Here's how the part is built. I have some questions about the finished solid (model axes, mm). A direction names the side the tool comes from. Coordinates: 2 decimals unless noted, no trailing zeros. Loops run counter-clockwise (first coordinate to the right, second up) from the corner with the lowest first, then second, coordinate; pieces in that order, holes last. Notation, with made-up numbers: M 14.25,75 L 19.25,75 A26 cw 19.25,93 Z; hole C 11,16.25 d4. An arc over 180 degrees is marked long. Use CSV: the item, a comma, the result in double quotes. Start each with the question number.
Q1. If we section it at A-A (x = -9): Please give me the cut outline in (y, z).
Q2. If we section it at C-C (y = 4.25): Please give me the cut outline in (x, z).
Q3. If we mould it in two halves opening along X, with no side actions, what happens to faces 1 (the cylindrical face through (-70.885, 26.549, -133.04)), 2 (the flat face through (-80, 15, -69)), 3 (the flat face through (-39, 27.5, -71))? For each: +X half, -X half, draft (parallel to the pull), parting line (faces both ways), or undercut.
Q4. Please list where these lines run through material, in increasing order: probe 1 along Y at (x, z) = (-46.5, -73); probe 2 along X at (y, z) = (25, -132.5); probe 3 along Z at (x, y) = (-9.5, 13). Write a range as [from, to].
Q5. For pin 1 Ø12 at (y, z) = (13.5, -49.5) entering from +X; pin 2 Ø2.5 at (x, z) = (-74.5, -131) entering from +Y, each with a flat end and sliding along its axis, tell me the tip position at first contact or that it passes through.
Q6. If we section it at D-D (x = -75): Please give me the cut outline in (y, z).
Q7. Which directions (+Z, -Z, +X, -X, +Y, -Y) give clear straight access to the entire face, cutting with the end or side of a thin tool? Please do faces 4 (the flat face through (-38, 15, -137.5)), 5 (the flat face through (-40, 30, -71)), 6 (the flat face through (-75, 23, -8)).
Q8. If we section it at B-B (z = -132.5): Please give me the cut outline in (x, y), and give its area (3 significant figures).
from build123d import *

# Parameters (mm, degrees)
SKETCH1_W           = 81
SKETCH1_H           = 140
BOSS_EXTRUDE2_DEPTH = 30
SKETCH3_R           = 4.15
CUT_EXTRUDE2_DEPTH  = 7
SHELL1_START        = 2.5
SHELL1_DEPTH        = 25
SHELL1_2_DEPTH      = 18


# Read off the part's stored shape, not the designer's step: Shell1
with BuildPart() as part:
    # Sketch1 → Boss-Extrude2 (new body)
    with BuildSketch(Plane(origin=(0, 0, 0), x_dir=(1, 0, 0), z_dir=(0, 1, 0))):
        with Locations((-39.5, 70)):
            Rectangle(SKETCH1_W, SKETCH1_H)
    extrude(amount=BOSS_EXTRUDE2_DEPTH)

    # Sketch3 → Cut-Extrude2 (cut)
    with BuildSketch(Plane(origin=(0, 30, 0), x_dir=(1, 0, 0), z_dir=(0, 1, 0))):
        with Locations(Location((-75, 7.5, 0), (0, 0, 270))):
            Circle(SKETCH3_R)
        with Locations(Location((-75, 132.5, 0), (0, 0, 270))):
            Circle(SKETCH3_R)
    extrude(amount=-CUT_EXTRUDE2_DEPTH, mode=Mode.SUBTRACT)

    # Shell1 outline → Shell1 (cut)
    with BuildSketch(Plane(origin=(0, 0, 0), x_dir=(1, 0, 0), z_dir=(0, 1, 0)).offset(SHELL1_START)):
        with BuildLine():
            Line((1, 137.5), (-70.615652842, 137.5))
            ThreePointArc((-70.615652842, 137.5), (-69.339940487, 129.009122415), (-77.5, 126.337816945))
            Line((-77.5, 126.337816945), (-77.5, 13.662183055))
            ThreePointArc((-77.5, 13.662183055), (-69.339940487, 10.990877585), (-70.615652842, 2.5))
            Line((-70.615652842, 2.5), (1, 2.5))
            Line((1, 2.5), (1, 137.5))
        make_face()
    extrude(amount=SHELL1_DEPTH, mode=Mode.SUBTRACT)

    # Shell1 2 outline → Shell1 2 (cut)
    with BuildSketch(Plane(origin=(0, 0, 0), x_dir=(1, 0, 0), z_dir=(0, 1, 0)).offset(SHELL1_START)):
        with BuildLine():
            Line((-70.615652842, 137.5), (-77.5, 137.5))
            Line((-77.5, 137.5), (-77.5, 126.337816945))
            ThreePointArc((-77.5, 126.337816945), (-69.339940487, 129.009122415), (-70.615652842, 137.5))
        make_face()
        with BuildLine():
            ThreePointArc((-70.615652842, 2.5), (-69.339940487, 10.990877585), (-77.5, 13.662183055))
            Line((-77.5, 13.662183055), (-77.5, 2.5))
            Line((-77.5, 2.5), (-70.615652842, 2.5))
        make_face()
    extrude(amount=SHELL1_2_DEPTH, mode=Mode.SUBTRACT)


solid = part.part
Results below:
1,outline,"M 0,-140 L 30,-140 L 30,0 L 0,0 Z; hole M 2.5,-137.5 L 27.5,-137.5 L 27.5,-2.5 L 2.5,-2.5 Z"
2,outline,"M -80,-140 L 1,-140 L 1,-137.5 L -77.5,-137.5 L -77.5,-2.5 L 1,-2.5 L 1,0 L -80,0 Z"
3,face 1,"undercut"
3,face 2,"-X half"
3,face 3,"draft"
4,probe 1,"[0, 2.5], [27.5, 30]"
4,probe 2,"[-80, -79.15], [-70.85, -68.35]"
4,probe 3,"[-140, -137.5], [-2.5, 0]"
5,pin 1,"x = -77.5"
5,pin 2,"y = 23"
6,outline,"M 0,-140 L 30,-140 L 30,-136.65 L 23,-136.65 L 23,-128.35 L 30,-128.35 L 30,-11.65 L 23,-11.65 L 23,-3.35 L 30,-3.35 L 30,0 L 0,0 Z; hole M 2.5,-137.5 L 20.5,-137.5 L 20.5,-125.85 L 27.5,-125.85 L 27.5,-14.15 L 20.5,-14.15 L 20.5,-2.5 L 2.5,-2.5 Z"
7,face 4,"+X"
7,face 5,"+Z, -Z, +X, -X, +Y"
7,face 6,"+Y"
8,outline,"M -80,0 L 1,0 L 1,2.5 L -77.5,2.5 L -77.5,20.5 L -68.35,20.5 L -68.35,27.5 L 1,27.5 L 1,30 L -70.85,30 L -70.85,23 L -79.15,23 L -79.15,30 L -80,30 Z"
8,area,"473 mm^2"
